Design review of the part shown in the three views and the two pictorial views. Dimensions are in mm from the part's minimum x, y and z. A direction names the side the tool comes from. Round coordinates to 2 decimals unless told otherwise and drop trailing zeros. Order: outer loops, then holes, each group sorted by start corner. A loop starts at its lowest first (then second) coordinate and runs counter-clockwise, first axis right, second up. Notation, with made-up numbers: (56, 68) -> (114, 68) arc R28 cw to (114, 98) -> close; hole circle Ø5 at (14.5, -13). An arc over 180 degrees is marked (long way). Put each result on its own line as item: value. Start each with the question number.
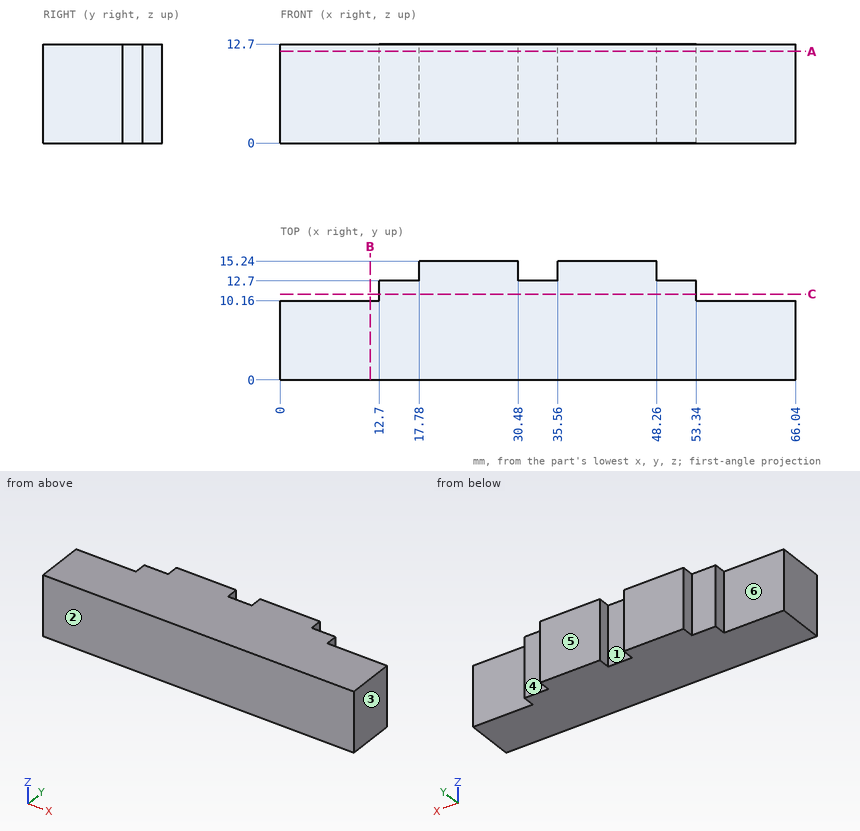
Q1. Take a section at A-A on z = 11.75. Give the boundary of the cut face in (x, y), and give its area (3 significant figures).
Q2. Wall thickness on probe 1 along X at (y, z) = (13, 11.5); probe 2 along X at (y, z) = (12, 3.5); probe 3 along Y at (x, z) = (53, 1): over which ranges is each line inside the solid? List them lowest first. Write a range as [from, to].
Q3. Take a section at C-C on y = 11. Give the boundary of the cut face in (x, z), and give its area (3 significant figures).
Q4. For the marked faces 4, 5 and 6, list the 3-axis set-ups (+Z, -Z, +X, -X, +Y, -Y) from which the entire face can be reached by the end or side of a thin tool; tool diameter is ignored.
Q5. Take a section at B-B on x = 11.5. Give the boundary of the cut face in (y, z), and give its area (3 significant figures).
Q6. Draft analysis for pull direction X (two halves, no side actions). For the marked faces 1, 2 and 3, state which applies: +X half, -X half, draft (parallel to the pull), parting line (faces both ways), or undercut.
Q7. Clearance check with flat-ended pins moving along their axes: pin 1 Ø6 at (x, y) = (43, 2) entering from -Z; pin 2 Ø2 at (y, z) = (12, 5.5) entering from +X; pin 3 Ø0.8 at (y, z) = (13.5, 7) entering from +X; pin 4 Ø1.5 at (x, z) = (14.5, 9.5) entering from +Y. State where each tip first meets the part, or that it passes through.
Calculated:
1. outline: (0, 0) -> (66.04, 0) -> (66.04, 10.16) -> (53.34, 10.16) -> (53.34, 12.7) -> (48.26, 12.7) -> (48.26, 15.24) -> (35.56, 15.24) -> (35.56, 12.7) -> (30.48, 12.7) -> (30.48, 15.24) -> (17.78, 15.24) -> (17.78, 12.7) -> (12.7, 12.7) -> (12.7, 10.16) -> (0, 10.16) -> close
1. area: 839 mm²
2. probe 1: x = [17.78, 30.48], [35.56, 48.26]
2. probe 2: x = [12.7, 53.34]
2. probe 3: y = [0, 12.7]
3. outline: (12.7, 0) -> (53.34, 0) -> (53.34, 12.7) -> (12.7, 12.7) -> close
3. area: 516 mm²
4. face 4: +Z, -Z, +X, +Y
4. face 5: +Z, -Z, +X, -X, +Y
4. face 6: +Z, -Z, -X, +Y
5. outline: (0, 0) -> (10.16, 0) -> (10.16, 12.7) -> (0, 12.7) -> close
5. area: 129 mm²
6. face 1: undercut
6. face 2: draft
6. face 3: +X half
7. pin 1: stops at z = 0
7. pin 2: stops at x = 53.34
7. pin 3: stops at x = 48.26
7. pin 4: stops at y = 12.7
